Geometry check sheet. Reference: the model listing, model coordinates, mm. A direction names the side the tool comes from. Coordinates: 2 decimals unless noted, no trailing zeros. Write each loop counter-clockwise with the first axis right and the second up, starting at its lowest first coordinate (ties: lowest second). Pieces come first, ordered by that corner, then holes. Notation, with made-up numbers: (64.5, 8.25) -> (115.5, 8.25) arc R10 ccw to (115.5, 14.25) -> close; hole circle Ø8 at (-20.75, -31). An arc over 180 degrees is marked (long way). Answer in a Markdown table with one row per item. Add a question column.
Q1. Section check A-A, the plane x = 20. Record the boundary of the cut face in (y, z).
Q2. Release check for a two-part mould opening along X. For faces 1 (the face through (10, -9.6, -10)), 2 (the face through (15.5, -20, -16)), 3 (the face through (5, -5, -12)) record: pulls with the +X half, pulls with the -X half, needs draft (parallel to the pull), parting line crosses it, or undercut.
Q3. Section check D-D, the plane z = -13.5. Record the boundary of the cut face in (x, y), and give its area (3 significant figures).
Q4. Section check B-B, the plane z = 3.5. Record the boundary of the cut face in (x, y).
Q5. Thickness scan on line 1 (Z direction, x = 20, y = -6); line 2 (X direction, y = -35.8, z = 3.45); line 3 (Y direction, x = 5, z = -15.75). Record the ranges inside material, lowest first.
Q6. Section check C-C, the plane y = -7.5. Record the boundary of the cut face in (x, z), and give its area (3 significant figures).
Q7. Tool access check on faces 4 (the face through (7, -25.2, -16)), 5 (the face through (-3.5, -7, 5)), 6 (the face through (-0.5, -20, -16)), 7 (the face through (22.5, -7, -7)), 8 (the face through (-3, -7, 4)). Record the directions out of +Z, -Z, +X, -X, +Y, -Y that give a thin tool (end or side, any length) a straight path to the whole face; none if there is none.
Q8. Gauge pin test, flat ends, axial feed: P1, Ø3, axis at x = 20, z = -13.5, coming from the +Y side; P2, Ø1, axis at x = -12.5, y = -8.5, coming from the +Z side; P3, Ø4, axis at x = -20, z = -2.5, coming from the +Y side; P4, Ø7.5, axis at x = 6, z = -12.5, coming from the -Y side. Record the tip position at first contact, or that the pin passes through.
```python
from build123d import *

# Parameters (mm, degrees)
CYLINDER043_R           = 1.75
CYLINDER043_DEPTH       = 44
CYLINDER043_ROLL_ANGLE  = 90
CYLINDER045_R           = 6
CYLINDER045_DEPTH       = 34
CYLINDER045_ROLL_ANGLE  = 90
BOX078_W                = 17
BOX078_H                = 17.6
BOX078_DEPTH            = 12
CYLINDER046_R           = 1.75
CYLINDER046_DEPTH       = 44
CYLINDER046_ROLL_ANGLE  = 90
BOX082_W                = 2
BOX082_H                = 24.6
BOX082_DEPTH            = 16
CYLINDER040_R           = 1.75
CYLINDER040_DEPTH       = 44
CYLINDER040_ROLL_ANGLE  = 90
CYLINDER047_R           = 1.75
CYLINDER047_DEPTH       = 21
CYLINDER047_PITCH_ANGLE = 90
CYLINDER052_R           = 1.5
CYLINDER052_DEPTH       = 42
BOX088_W                = 42
BOX088_H                = 3
BOX088_DEPTH            = 3
CYLINDER044_R           = 1.75
CYLINDER044_DEPTH       = 44
CYLINDER044_ROLL_ANGLE  = 90
BOX075_W                = 26
BOX075_H                = 4.6
BOX075_DEPTH            = 25
BOX083_W                = 14
BOX083_H                = 4.6
BOX083_DEPTH            = 3
BOX086_W                = 8
BOX086_H                = 32.6
BOX086_DEPTH            = 3.5
BOX087_W                = 16
BOX087_H                = 20.6
BOX087_DEPTH            = 6.5
BOX079_W                = 5
BOX079_H                = 10.6
BOX079_DEPTH            = 25


with BuildPart() as cylinder_for_hole_9_groovemount_l004:
    # Cylinder043 → Cylinder043 (new body)
    with BuildSketch(Plane.XY):
        Circle(CYLINDER043_R)
    extrude(amount=CYLINDER043_DEPTH)


with BuildPart() as cylinder_for_hole_9_groovemount_l004_1:
    # Cylinder043 roll: moved
    add(cylinder_for_hole_9_groovemount_l004.part.rotate(Axis((0, 0, 0), (1, 0, 0)), CYLINDER043_ROLL_ANGLE))


with BuildPart() as cylinder_for_hole_9_groovemount_l004_2:
    # Cylinder043 placement: moved
    add(cylinder_for_hole_9_groovemount_l004_1.part.moved(Location((-20, 6, -2.5))))


with BuildPart() as jhead_hole001:
    # Cylinder045 → Cylinder045 (new body)
    with BuildSketch(Plane.XY):
        Circle(CYLINDER045_R)
    extrude(amount=CYLINDER045_DEPTH)


with BuildPart() as jhead_hole001_1:
    # Cylinder045 roll: moved
    add(jhead_hole001.part.rotate(Axis((0, 0, 0), (1, 0, 0)), CYLINDER045_ROLL_ANGLE))


with BuildPart() as jhead_hole001_2:
    # Cylinder045 placement: moved
    add(jhead_hole001_1.part.moved(Location((7.5, 0, -4))))


with BuildPart() as jhead_retention_plate_slide_in_hole001:
    # Box078 → Box078 (new body)
    with BuildSketch(Plane(origin=(-9.5, -14.6, -10), x_dir=(1, 0, 0), z_dir=(0, 0, 1))):
        with Locations((8.5, 8.8)):
            Rectangle(BOX078_W, BOX078_H)
    extrude(amount=BOX078_DEPTH)


with BuildPart() as cylinder_for_hole_4_motherboard004:
    # Cylinder046 → Cylinder046 (new body)
    with BuildSketch(Plane.XY):
        Circle(CYLINDER046_R)
    extrude(amount=CYLINDER046_DEPTH)


with BuildPart() as cylinder_for_hole_4_motherboard004_1:
    # Cylinder046 roll: moved
    add(cylinder_for_hole_4_motherboard004.part.rotate(Axis((0, 0, 0), (1, 0, 0)), CYLINDER046_ROLL_ANGLE))


with BuildPart() as cylinder_for_hole_4_motherboard004_2:
    # Cylinder046 placement: moved
    add(cylinder_for_hole_4_motherboard004_1.part.moved(Location((20, 6, -13.5))))


with BuildPart() as retention_hexagon_head_slide_in_hole:
    # Box082 → Box082 (new body)
    with BuildSketch(Plane(origin=(-3.5, -14.6, -12), x_dir=(1, 0, 0), z_dir=(0, 0, 1))):
        with Locations((1, 12.3)):
            Rectangle(BOX082_W, BOX082_H)
    extrude(amount=BOX082_DEPTH)


with BuildPart() as cylinder_for_hole_3_motherboard003:
    # Cylinder040 → Cylinder040 (new body)
    with BuildSketch(Plane.XY):
        Circle(CYLINDER040_R)
    extrude(amount=CYLINDER040_DEPTH)


with BuildPart() as cylinder_for_hole_3_motherboard003_1:
    # Cylinder040 roll: moved
    add(cylinder_for_hole_3_motherboard003.part.rotate(Axis((0, 0, 0), (1, 0, 0)), CYLINDER040_ROLL_ANGLE))


with BuildPart() as cylinder_for_hole_3_motherboard003_2:
    # Cylinder040 placement: moved
    add(cylinder_for_hole_3_motherboard003_1.part.moved(Location((-20, 6, -13.5))))


with BuildPart() as f_30x30_fan_hole:
    # Cylinder047 → Cylinder047 (new body)
    with BuildSketch(Plane.XY):
        Circle(CYLINDER047_R)
    extrude(amount=CYLINDER047_DEPTH)


with BuildPart() as f_30x30_fan_hole_1:
    # Cylinder047 pitch: moved
    add(f_30x30_fan_hole.part.rotate(Axis((0, 0, 0), (0, 1, 0)), CYLINDER047_PITCH_ANGLE))


with BuildPart() as f_30x30_fan_hole_2:
    # Cylinder047 placement: moved
    add(f_30x30_fan_hole_1.part.moved(Location((-24, -10, 11))))


with BuildPart() as extruder_screw_r:
    # Cylinder052 → Cylinder052 (new body)
    with BuildSketch(Plane(origin=(16.8, -35.8, -8), x_dir=(1, 0, 0), z_dir=(0, 0, 1))):
        Circle(CYLINDER052_R)
    extrude(amount=CYLINDER052_DEPTH)


with BuildPart() as fastener_hole:
    # Box088 → Box088 (new body)
    with BuildSketch(Plane(origin=(-21.5, -28.2, -17.5), x_dir=(1, 0, 0), z_dir=(0, 0, 1))):
        with Locations((21, 1.5)):
            Rectangle(BOX088_W, BOX088_H)
    extrude(amount=BOX088_DEPTH)


with BuildPart() as hexagon_retention_block_holes:
    # Cylinder044 → Cylinder044 (new body)
    with BuildSketch(Plane.XY):
        Circle(CYLINDER044_R)
    extrude(amount=CYLINDER044_DEPTH)


with BuildPart() as hexagon_retention_block_holes_1:
    # Cylinder044 roll: moved
    add(hexagon_retention_block_holes.part.rotate(Axis((0, 0, 0), (1, 0, 0)), CYLINDER044_ROLL_ANGLE))


with BuildPart() as hexagon_retention_block_holes_2:
    # Cylinder044 placement: moved
    add(hexagon_retention_block_holes_1.part.moved(Location((20, 6, -2.5))))

    # Fusion020: union cylinder for hole 9 - Groovemount L004, jhead hole001, jhead retention plate slide in hole001, cylinder for hole 4 - Motherboard004, retention hexagon head slide in hole, cylinder for hole 3 - Motherboard003, 30x30 fan hole, extruder screw  R, fastener hole
    add(cylinder_for_hole_9_groovemount_l004_2.part)
    add(jhead_hole001_2.part)
    add(jhead_retention_plate_slide_in_hole001.part)
    add(cylinder_for_hole_4_motherboard004_2.part)
    add(retention_hexagon_head_slide_in_hole.part)
    add(cylinder_for_hole_3_motherboard003_2.part)
    add(f_30x30_fan_hole_2.part)
    add(extruder_screw_r.part)
    add(fastener_hole.part)


with BuildPart() as jhead_retention_plate_body001:
    # Box075 → Box075 (new body)
    with BuildSketch(Plane(origin=(-3.5, -9.6, -19), x_dir=(1, 0, 0), z_dir=(0, 0, 1))):
        with Locations((13, 2.3)):
            Rectangle(BOX075_W, BOX075_H)
    extrude(amount=BOX075_DEPTH)


with BuildPart() as fan_bracket_retention_plate_joint:
    # Box083 → Box083 (new body)
    with BuildSketch(Plane(origin=(-17.5, -9.6, -19), x_dir=(1, 0, 0), z_dir=(0, 0, 1))):
        with Locations((7, 2.3)):
            Rectangle(BOX083_W, BOX083_H)
    extrude(amount=BOX083_DEPTH)


with BuildPart() as motor_bracket_base_r:
    # Box086 → Box086 (new body)
    with BuildSketch(Plane(origin=(12.5, -40.2, 2.5), x_dir=(1, 0, 0), z_dir=(0, 0, 1))):
        with Locations((4, 16.3)):
            Rectangle(BOX086_W, BOX086_H)
    extrude(amount=BOX086_DEPTH)


with BuildPart() as motor_support:
    # Box087 → Box087 (new body)
    with BuildSketch(Plane(origin=(-0.5, -30.2, -19), x_dir=(1, 0, 0), z_dir=(0, 0, 1))):
        with Locations((8, 10.3)):
            Rectangle(BOX087_W, BOX087_H)
    extrude(amount=BOX087_DEPTH)


with BuildPart() as hexagon_retention_block_with_holes:
    # Box079 → Box079 (new body)
    with BuildSketch(Plane(origin=(-22.5, -15.6, -19), x_dir=(1, 0, 0), z_dir=(0, 0, 1))):
        with Locations((2.5, 5.3)):
            Rectangle(BOX079_W, BOX079_H)
    extrude(amount=BOX079_DEPTH)

    # Fusion021: union jhead retention plate body001, fan bracket retention plate joint, motor bracket base R, motor support
    add(jhead_retention_plate_body001.part)
    add(fan_bracket_retention_plate_joint.part)
    add(motor_bracket_base_r.part)
    add(motor_support.part)

    # Cut012: cut hexagon retention block holes
    add(hexagon_retention_block_holes_2.part, mode=Mode.SUBTRACT)


solid = hexagon_retention_block_with_holes.part
```
Calculated:
| question | item | result |
|---|---|---|
| 1 | outline | (-40.2, 2.5) -> (-9.6, 2.5) -> (-9.6, -0.75) -> (-5, -0.75) -> (-5, 6) -> (-40.2, 6) -> close; (-9.6, -19) -> (-5, -19) -> (-5, -15.25) -> (-9.6, -15.25) -> close; (-9.6, -11.75) -> (-5, -11.75) -> (-5, -4.25) -> (-9.6, -4.25) -> close |
| 2 | face 1 | undercut |
| 2 | face 2 | pulls with the +X half |
| 2 | face 3 | needs draft |
| 3 | outline | (-22.5, -15.6) -> (-21.75, -15.6) -> (-21.75, -5) -> (-22.5, -5) -> close; (-18.25, -15.6) -> (-17.5, -15.6) -> (-17.5, -5) -> (-18.25, -5) -> close; (-3.5, -9.6) -> (-0.5, -9.6) -> (-0.5, -30.2) -> (15.5, -30.2) -> (15.5, -9.6) -> (18.25, -9.6) -> (18.25, -5) -> (-3.5, -5) -> close; (21.75, -9.6) -> (22.5, -9.6) -> (22.5, -5) -> (21.75, -5) -> close |
| 3 | area | 449 mm² |
| 4 | outline | (-22.5, -15.6) -> (-17.5, -15.6) -> (-17.5, -5) -> (-22.5, -5) -> close; (-1.5, -9.6) -> (12.5, -9.6) -> (12.5, -40.2) -> (20.5, -40.2) -> (20.5, -9.6) -> (22.5, -9.6) -> (22.5, -5) -> (-1.5, -5) -> close; hole circle Ø3 at (16.8, -35.8) |
| 5 | line 1 | z = -19 to -15.25, -11.75 to -4.25, -0.75 to 6 |
| 5 | line 2 | x = 12.5 to 15.3, 18.3 to 20.5 |
| 5 | line 3 | y = -30.2 to -28.2, -25.2 to -5 |
| 6 | outline | (-22.5, -19) -> (22.5, -19) -> (22.5, 6) -> (-3.5, 6) -> (-3.5, 4) -> (-1.5, 4) -> (-1.5, 2) -> (7.5, 2) arc R6 cw to (7.5, -10) -> (-1.5, -10) -> (-1.5, -12) -> (-3.5, -12) -> (-3.5, -16) -> (-17.5, -16) -> (-17.5, 6) -> (-22.5, 6) -> close; hole circle Ø3.5 at (-20, -13.5); hole circle Ø3.5 at (-20, -2.5); hole circle Ø3.5 at (20, -13.5); hole circle Ø3.5 at (20, -2.5) |
| 6 | area | 582 mm² |
| 7 | face 4 | +X, -X |
| 7 | face 5 | +Z, +Y, -Y |
| 7 | face 6 | +Z, -Z, -Y |
| 7 | face 7 | +Z, -Z, +X, +Y, -Y |
| 7 | face 8 | +Y, -Y |
| 8 | P1 | passes through |
| 8 | P2 | stops at z = -16 |
| 8 | P3 | stops at y = -5 |
| 8 | P4 | stops at y = -30.2 |
